The listing builds one solid part. Answer for the finished solid, in the listing's coordinates (mm). A direction names the side the tool comes from. Give positions to 0.01 mm unless a question says otherwise; leave off trailing zeros. Loops run counter-clockwise (first coordinate to the right, second up) from the corner with the lowest first, then second, coordinate; pieces in that order, holes last.
Item 1: A tool of negligible diameter and unlimited length cuts with its end or side. For faces 1 (the face through (48.6, 24.3, 1.372)), 2 (the face through (48.933, 25.773, 0.281)), 3 (the face through (46.312, 39.964, 0.977)), from which of +Z, -Z, +X, -X, +Y, -Y can it reach the whole face along a straight path? Write none if from no direction.
Item 2: Consider line 1 along Z through (x, y) = (50.25, 28.5); line 2 along X through (y, z) = (39, 0.05); line 3 along Y through (x, z) = (50.5, 1.8). Determine where each line is inside the solid, lowest interval first.
Item 3: The mould has two halves that part along Y. Classify faces 4 (the face through (50.33, 25.59, 0.29)), 5 (the face through (49, 39, 0)), 6 (the face through (48.6, 24.3, 0.61)): pulls with the +Y half, pulls with the -Y half, needs draft (parallel to the pull), parting line crosses it, or undercut.
Item 4: Section A-A, the plane y = 39.5 is taken. Give the vertices of the cut face in (x, z).
Item 5: Each of these flat-tipped pins is pushed along its axis until it touches: pin 1 Ø4 at (x, y) = (45.5, 28) entering from +Z; pin 2 Ø2 at (x, y) = (46, 31) entering from +Z; pin 3 Ø0.7 at (x, y) = (50, 24.5) entering from +Z; pin 4 Ø0.9 at (x, y) = (49, 24) entering from -Z. Where does it stop, or does it pass through?
from build123d import *

# Parameters (mm, degrees)
SKETCH1_R           = 2.0955
BOSS_EXTRUDE1_DEPTH = 1.9812
FILLET1_R           = 0.762
SKETCH3_R           = 1.27
BOSS_EXTRUDE2_DEPTH = 4.6355
SKETCH5_W           = 0.830502785
SKETCH5_H           = 0.830502786
CUT_EXTRUDE1_DEPTH  = 3.81
CUT_EXTRUDE2_DEPTH  = 3.81
CIRPATTERN1_COUNT   = 4
FILLET3_R           = 0.254


with BuildPart() as part:
    # Sketch1 → Boss-Extrude1 (new body)
    with BuildSketch(Plane.XY):
        with BuildLine():
            Line((45.760103821, 50.326590864), (45.760103821, 46.618317867))
            Line((45.760103821, 46.618317867), (43.856665355, 46.618317867))
            Line((43.856665355, 46.618317867), (43.347103821, 39.150717867))
            ThreePointArc((43.347103821, 39.150717867), (44.016000174, 38.394427109), (44.848352407, 38.965905721))
            ThreePointArc((44.848352407, 38.965905721), (46.339305619, 39.960432804), (47.471727095, 38.571315385))
            Line((47.471727095, 38.571315385), (46.903103821, 27.974717867))
            ThreePointArc((46.903103821, 27.974717867), (47.275078209, 27.076692255), (48.173103821, 26.704717867))
            Line((48.173103821, 26.704717867), (50.12121108, 26.450717867))
            ThreePointArc((50.12121108, 26.450717867), (51.01744047, 26.560052876), (51.472746702, 27.339717867))
            Line((51.472746702, 27.339717867), (52.999103821, 49.708408747))
            ThreePointArc((52.999103821, 49.708408747), (49.552184435, 52.0384432), (45.760103821, 50.326590864))
        make_face()
        with Locations((49.189103821, 47.786717867)):
            Circle(SKETCH1_R, mode=Mode.SUBTRACT)
    extrude(amount=BOSS_EXTRUDE1_DEPTH)

    # Fillet1
    fillet1_edges = [part.edges().sort_by_distance(p)[0] for p in [
        (43.856665355, 46.618317867, 0.9906),
        (45.760103821, 46.618317867, 0.9906),
    ]]
    fillet(fillet1_edges, radius=FILLET1_R)

    # Sketch3 → Boss-Extrude2 (add)
    with BuildSketch(Plane(origin=(4.228879683, 32.434296092, 0), x_dir=(0.9916069999104432, -0.12928866047960397, 0), z_dir=(-0.12928866047960397, -0.9916069999104432, 0))):
        with Locations(Location((45.888507166, 0.9906, 0), (0, 0, 231.260575402))):
            Circle(SKETCH3_R)
    extrude(amount=BOSS_EXTRUDE2_DEPTH)

    # Sketch5 → Cut-Extrude1 (cut)
    with BuildSketch(Plane(origin=(3.629562097, 27.837701844, 0), x_dir=(0.9916069999104432, -0.129288660479604, 0), z_dir=(-0.129288660479604, -0.9916069999104432, 0))):
        with Locations((46.684758559, 1.786851393)):
            Rectangle(SKETCH5_W, SKETCH5_H)
    cut_extrude1 = extrude(amount=-CUT_EXTRUDE1_DEPTH, mode=Mode.SUBTRACT)

    # Sketch6 → Cut-Extrude2 (cut)
    with BuildSketch(Plane(origin=(45.881167188, -5.982122602, 0), x_dir=(0, 0, -1), z_dir=(0.9916069999104432, -0.129288660479604, 0))):
        Polygon((-1.3716, 28.073321232), (-2.2606, 29.978321232), (-2.2606, 28.073321232), align=None)
    cut_extrude2 = extrude(amount=-CUT_EXTRUDE2_DEPTH, mode=Mode.SUBTRACT)

    # CirPattern1: Cut-Extrude1, Cut-Extrude2 ×4 about axis
    cirpattern1_axis = Axis((45.503364921, -5.932863623, 0.9906), (0.1292886604796056, 0.991606999910443, 0))
    add([cut_extrude1.rotate(cirpattern1_axis, i * 360 / CIRPATTERN1_COUNT) for i in range(1, CIRPATTERN1_COUNT)], mode=Mode.SUBTRACT)
    add([cut_extrude2.rotate(cirpattern1_axis, i * 360 / CIRPATTERN1_COUNT) for i in range(1, CIRPATTERN1_COUNT)], mode=Mode.SUBTRACT)

    # Fillet3
    # the kernel refuses this fillet: 0.254 mm, written as the material it adds along each edge
    with BuildSketch(Plane(origin=(48.314504429, 26.686281636, 1.9812), x_dir=(0.1292886604796056, 0.9916069999104429, 0), z_dir=(0.991606999910443, -0.1292886604796056, -1.1175710787249272e-14))) as fillet3_piece_1_section:
        with BuildLine():
            CenterArc((FILLET3_R, FILLET3_R), FILLET3_R, 180, 90)
            Line((0, FILLET3_R), (0, 0))
            Line((0, 0), (FILLET3_R, 0))
        make_face()
    fillet3_piece_1 = extrude(amount=2.859479965, mode=Mode.PRIVATE)
    fillet3_piece_1 = fillet3_piece_1 & Plane(origin=(49.739170081, 26.554548895, 0.9906), x_dir=(-0.6205273463723372, 0.08090619510621488, -0.7799999999984234), z_dir=(0.12928866047960397, 0.9916069999104432, 0)) * Cylinder(1.27, 7, mode=Mode.PRIVATE)
    add(fillet3_piece_1)
    with BuildSketch(Plane(origin=(51.149984779, 26.316583302, 0), x_dir=(0.12928866047960436, 0.9916069999104431, 0), z_dir=(-0.9916069999104432, 0.12928866047960438, 1.2608297213769615e-12))) as fillet3_piece_2_section:
        with BuildLine():
            CenterArc((FILLET3_R, FILLET3_R), FILLET3_R, 180, 90)
            Line((0, FILLET3_R), (0, 0))
            Line((0, 0), (FILLET3_R, 0))
        make_face()
    fillet3_piece_2 = extrude(amount=2.859479965, mode=Mode.PRIVATE)
    fillet3_piece_2 = fillet3_piece_2 & Plane(origin=(49.73917008, 26.554548887, 0.9906), x_dir=(-0.6205273463723372, 0.08090619510621488, -0.7799999999984234), z_dir=(0.12928866047960397, 0.9916069999104432, 0)) * Cylinder(1.27, 7, mode=Mode.PRIVATE)
    add(fillet3_piece_2)


solid = part.part
Worked answers:
1. face 1: +Z, -X
1. face 2: -Z, -X
1. face 3: +Z, -Z
2. line 1: z = 0 to 1.98
2. line 2: x = 43.36 to 44.86, 47.42 to 52.27
2. line 3: y = 25.57 to 46.15, 49.42 to 51.85
3. face 4: pulls with the -Y half
3. face 5: needs draft
3. face 6: undercut
4. outline: (43.37, 0) - (45.12, 0) - (45.12, 1.98) - (43.37, 1.98) - close; (47.16, 0) - (52.3, 0) - (52.3, 1.98) - (47.16, 1.98) - close
5. pin 1: stops at z = 1.98
5. pin 2: passes through
5. pin 3: stops at z = 2.25
5. pin 4: stops at z = -0.28
